from build123d import *

# Parameters (mm, degrees)
F0_W     = 35
F0_H     = 23
F1_DEPTH = 29
F2_W     = 49
F2_H     = 25
F2_W_2   = 35
F2_H_2   = 23
F3_DEPTH = 15


with BuildPart() as f1:
    # F0 (on Top) → F1 (new body)
    with BuildSketch(Plane.XY):
        with Locations((6.9202957675, 8.4343513213)):
            Rectangle(F0_W, F0_H)
    extrude(amount=F1_DEPTH)

    # F2 (on face) → F3 (join)
    with BuildSketch(Plane.XY.offset(29)):
        with Locations((6.9202957675, 8.4343513213)):
            Rectangle(F2_W, F2_H)
        with Locations((6.9202957675, 8.4343513213)):
            Rectangle(F2_W_2, F2_H_2, mode=Mode.SUBTRACT)
        with Locations((6.9202957675, 8.4343513213)):
            Rectangle(F2_W_2, F2_H_2)
    extrude(amount=F3_DEPTH)


solid = f1.part
The listing builds one solid part. Answer for the finished solid, in the listing's coordinates (mm). A direction names the side the tool comes from. Coordinates: 2 decimals unless noted, no trailing zeros. Write each loop counter-clockwise with the first axis right and the second up, starting at its lowest first coordinate (ties: lowest second). Pieces come first, ordered by that corner, then holes. Notation, with made-up numbers: (88, 47.25) - (140, 47.25) arc R22 cw to (140, 67.25) - close; hole circle Ø5 at (-28.75, 14.25). An arc over 180 degrees is marked (long way). Return JSON: item names as keys, results as strings.
1. The part is cut by section B-B on y = 14. Determine the outline of the cut face in (x, z), then the cut area to 3 significant figures.
Final values:
{"outline": "(-17.58, 29) - (-10.58, 29) - (-10.58, 0) - (24.42, 0) - (24.42, 29) - (31.42, 29) - (31.42, 44) - (-17.58, 44) - close", "area": "1,750 mm^2"}
2. The part is cut by section C-C on z = 3. Determine the outline of the cut face in (x, y).
Final values:
{"outline": "(-10.58, -3.07) - (24.42, -3.07) - (24.42, 19.93) - (-10.58, 19.93) - close"}
3. The part is cut by section A-A on x = 0.5. Determine the outline of the cut face in (y, z).
Final values:
{"outline": "(-4.07, 29) - (-3.07, 29) - (-3.07, 0) - (19.93, 0) - (19.93, 29) - (20.93, 29) - (20.93, 44) - (-4.07, 44) - close"}
4. The part is cut by section D-D on x = 25.5. Determine the outline of the cut face in (y, z), then the cut area to 3 significant figures.
Final values:
{"outline": "(-4.07, 29) - (20.93, 29) - (20.93, 44) - (-4.07, 44) - close", "area": "375 mm^2"}
5. Consider line 1 along Y through (x, z) = (10, 24); line 2 along X through (y, z) = (14.5, 18.5); line 3 along Z through (x, y) = (25, 14). Determine where each line is inside the solid, lowest interval first.
Final values:
{"line 1": "-3.07 to 19.93", "line 2": "-10.58 to 24.42", "line 3": "29 to 44"}
6. Which of the six approach directions +Z, -Z, +X, -X, +Y, -Y give full straight-line access (tool end or side, diameter ignored) to faces 1 (the face through (7, -3.066, 14)), 2 (the face through (-10.58, 8, 14)), 3 (the face through (24.42, 8, 14))?
Final values:
{"face 1": "-Z, +X, -X, -Y", "face 2": "-Z, -X, +Y, -Y", "face 3": "-Z, +X, +Y, -Y"}
7. Each of these flat-tipped pins is pushed along its axis until it touches: pin 1 Ø3 at (x, z) = (-5, 10) entering from +Y; pin 2 Ø2 at (x, z) = (3, 26) entering from -Y; pin 3 Ø4 at (y, z) = (7, 21) entering from +X. Where does it stop, or does it pass through?
Final values:
{"pin 1": "y = 19.93", "pin 2": "y = -3.07", "pin 3": "x = 24.42"}
